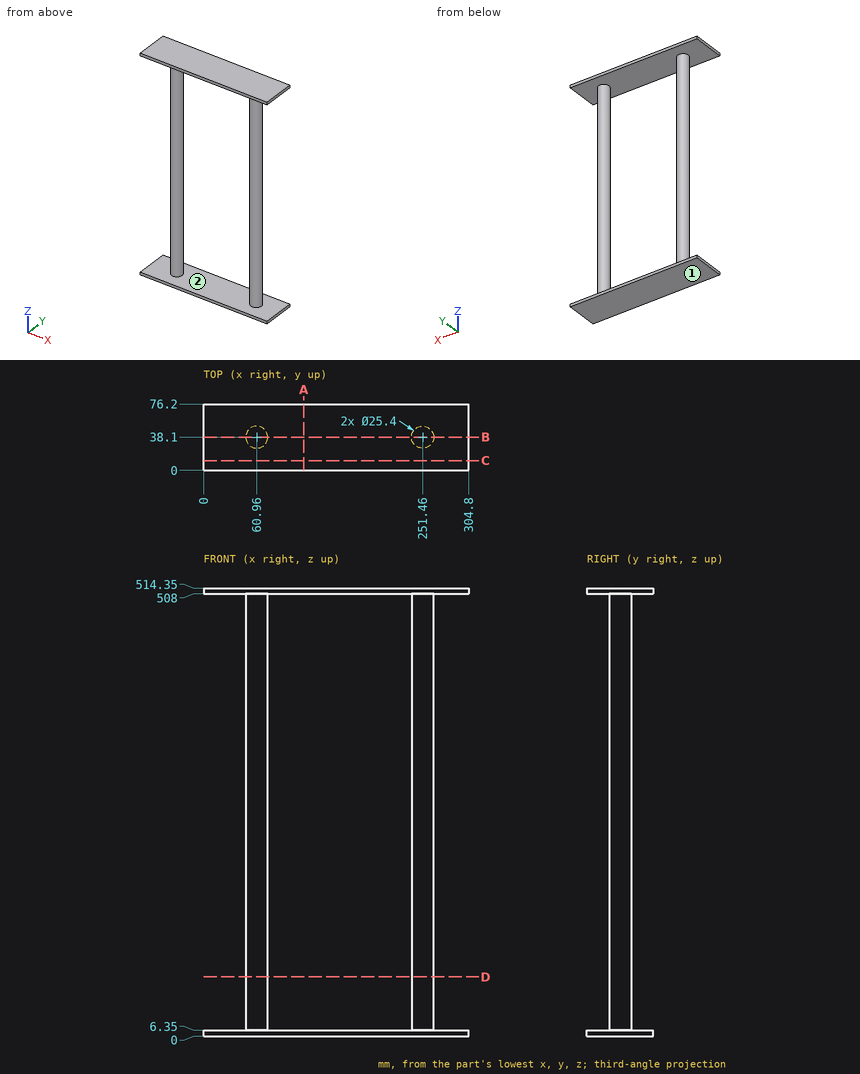
Input: dimensioned drawing with shaded views. Units: mm. Origin: part minimum x, y, z. Give positions to 0.01 mm unless a question says otherwise; leave off trailing zeros. Write each loop counter-clockwise with the first axis right and the second up, starting at its lowest first coordinate (ties: lowest second). Pieces come first, ordered by that corner, then holes.
Q1. Section A-A, the plane x = 115. Output: boundary loops of the cut face in (y, z).
Q2. Pull-direction query (X, two-part tool) for the marked faces 1 and 2; classes: pulls with the +X half, pulls with the -X half, needs draft (parallel to the pull), parting line crosses it, or undercut.
Q3. Material intervals for probe 1 along Z at (x, y) = (248.5, 10); probe 2 along X at (y, z) = (36.5, 153); probe 3 along X at (y, z) = (33.5, 86.5), sorted ascending.
Q4. Section C-C, the plane y = 11. Output: boundary loops of the cut face in (x, z), plus the area to 3 significant figures.
Q5. Section B-B, the plane y = 38.1. Output: boundary loops of the cut face in (x, z), plus the area to 3 significant figures.
Q6. Section D-D, the plane z = 68. Output: boundary loops of the cut face in (x, y), plus the area to 3 significant figures.
Filled in:
1. outline: (0, 0) - (76.2, 0) - (76.2, 6.35) - (0, 6.35) - close; (0, 508) - (76.2, 508) - (76.2, 514.35) - (0, 514.35) - close
2. face 1: needs draft
2. face 2: undercut
3. probe 1: z = 0 to 6.35, 508 to 514.35
3. probe 2: x = 48.36 to 73.56, 238.86 to 264.06
3. probe 3: x = 49.12 to 72.8, 239.62 to 263.3
4. outline: (0, 0) - (304.8, 0) - (304.8, 6.35) - (0, 6.35) - close; (0, 508) - (304.8, 508) - (304.8, 514.35) - (0, 514.35) - close
4. area: 3,870 mm2
5. outline: (0, 0) - (304.8, 0) - (304.8, 6.35) - (264.16, 6.35) - (264.16, 508) - (304.8, 508) - (304.8, 514.35) - (0, 514.35) - (0, 508) - (48.26, 508) - (48.26, 6.35) - (0, 6.35) - close; hole (73.66, 6.35) - (238.76, 6.35) - (238.76, 508) - (73.66, 508) - close
5. area: 29,400 mm2
6. outline: circle Ø25.4 at (60.96, 38.1); circle Ø25.4 at (251.46, 38.1)
6. area: 1,010 mm2
